Geometry: final body of the model. Coordinates: model frame, mm. Coordinates: 2 decimals unless noted, no trailing zeros. Order: outer loops, then holes, each group sorted by start corner. A loop starts at its lowest first (then second) coordinate and runs counter-clockwise, first axis right, second up. Notation, with made-up numbers: (63.5, 54) -> (100.5, 54) arc R8 cw to (100.5, 68) -> close; hole circle Ø9 at (-38.75, 42). An arc over 180 degrees is marked (long way). Answer in a Markdown table with one row per item. Add a question column.
1) Contact query for flat-ended pins moving along their axis: P1, Ø3, axis at x = 22, z = 12, coming from the -Y side; P2, Ø12, axis at x = 5.5, z = 12.5, coming from the +Y side; P3, Ø10, axis at x = -13.5, z = 6, coming from the +Y side. Output: stop coordinate, or through.
2) Section query A-A on y = 1. Return the cut outline in (x, z) (3 decimals), then the cut area to 3 significant figures.
3) Ray query, line 1 (Z direction, x = 16, y = -20.5) (3 decimals); line 2 (Y direction, x = -30, z = 0); line 3 (Y direction, x = -29.4, z = 0). Return the intervals inside material, ascending. Write a range as from..to.
4) Section query C-C on z = 0. Return the cut outline in (x, y).
5) Section query B-B on x = -20. Return the cut outline in (y, z) (3 decimals).
6) Section query D-D on z = 10.5. Return the cut outline in (x, y).
```python
from build123d import *

# Parameters (mm, degrees)
BOSS_EXTRUDE1_DEPTH       = 15.875
SKETCH2_W                 = 19.05
SKETCH2_H                 = 79.375
CUT_EXTRUDE1_DEPTH        = 12.7
FILLET1_R                 = 3.175
F_8_CLEARANCE_HOLE1_D     = 4.4958
F_8_CLEARANCE_HOLE1_DEPTH = 16.51
F_8_CLEARANCE_HOLE1_TIP   = 1.350674586
F_8_32_TAPPED_HOLE1_D     = 3.4544


with BuildPart() as part:
    # Sketch1 → Boss-Extrude1 (new, symmetric)
    with BuildSketch(Plane.XY):
        Polygon((-32.328922036, 32.328922036), (-32.328922036, 23.348665915), (27.838793975, -36.819050096), (32.328922036, -32.328922036), align=None)
    extrude(amount=BOSS_EXTRUDE1_DEPTH, both=True)

    # Sketch2 → Cut-Extrude1 (cut)
    with BuildSketch(Plane(origin=(0, 0, 0), x_dir=(0, 0, -1), z_dir=(0.7071067811865461, 0.707106781186549, 0))):
        with Locations((0, -2.3495)):
            Rectangle(SKETCH2_W, SKETCH2_H)
    extrude(amount=-CUT_EXTRUDE1_DEPTH, mode=Mode.SUBTRACT)

    # Fillet1
    fillet1_edges = [part.edges().sort_by_distance(p)[0] for p in [
        (27.47958373, -31.969711791, 9.525),
        (-28.647017026, 24.156888966, 9.525),
        (-28.647017026, 24.156888966, -9.525),
        (27.47958373, -31.969711791, -9.525),
    ]]
    fillet(fillet1_edges, radius=FILLET1_R)

    # #8 Clearance Hole1
    with Locations(Plane(origin=(29.724647761, -29.724647761, 0), x_dir=(0, 0, 1), z_dir=(-0.7071067811865489, 0.7071067811865462, 0))):
        with Locations((0, -3.175)):
            Hole(F_8_CLEARANCE_HOLE1_D / 2, depth=F_8_CLEARANCE_HOLE1_DEPTH)
            with Locations((0, 0, -(F_8_CLEARANCE_HOLE1_DEPTH + F_8_CLEARANCE_HOLE1_TIP / 2))):  # 118° drill point
                Cone(0, F_8_CLEARANCE_HOLE1_D / 2, F_8_CLEARANCE_HOLE1_TIP, mode=Mode.SUBTRACT)

    # #8-32 Tapped Hole1 (through all)
    with Locations(Plane.ZY.offset(32.328922036)):
        with Locations((0, 25.978922036)):
            Hole(F_8_32_TAPPED_HOLE1_D / 2)


solid = part.part
```
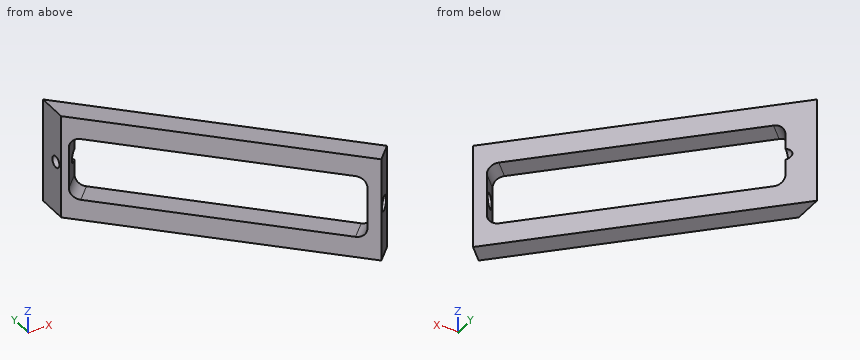
Result:
| question | item | result |
|---|---|---|
| 1 | P1 | y = -32.48 |
| 1 | P2 | y = 0.5 |
| 1 | P3 | y = 17.05 |
| 2 | outline | (-9.98, -15.875) -> (-1, -15.875) -> (-1, -9.525) -> (-9.98, -9.525) -> close; (-9.98, 9.525) -> (-1, 9.525) -> (-1, 15.875) -> (-9.98, 15.875) -> close |
| 2 | area | 114 mm2 |
| 3 | line 1 | -15.875..-9.525, 9.525..15.875 |
| 3 | line 2 | 22.8..24.25, 27.71..30 |
| 3 | line 3 | 23.4..24.25, 27.71..29.4 |
| 4 | outline | (-32.33, 23.35) -> (-30.89, 21.91) -> (-28.55, 24.25) -> (-32.33, 24.25) -> close; (-32.33, 27.71) -> (-27.71, 27.71) -> (-32.33, 32.33) -> close; (25.23, -34.21) -> (27.84, -36.82) -> (28.49, -36.16) -> (25.89, -33.56) -> close; (29.07, -30.38) -> (31.67, -32.98) -> (32.33, -32.33) -> (29.72, -29.72) -> close |
| 5 | outline | (11.02, -15.875) -> (20, -15.875) -> (20, -9.525) -> (11.02, -9.525) -> close; (11.02, 9.525) -> (20, 9.525) -> (20, 15.875) -> (11.02, 15.875) -> close |
| 6 | outline | (-32.33, 23.35) -> (27.84, -36.82) -> (32.33, -32.33) -> (-32.33, 32.33) -> close |
